```python
from build123d import *

# Parameters (mm, degrees)
SKETCH1_W           = 60
SKETCH1_H           = 100
BOSS_EXTRUDE1_DEPTH = 30
SKETCH2_W           = 60
SKETCH2_H           = 100
BOSS_EXTRUDE2_DEPTH = 30
SKETCH3_W           = 20
SKETCH3_H           = 30
BOSS_EXTRUDE3_DEPTH = 30
SKETCH4_W           = 1.6
SKETCH4_H           = 3
BOSS_EXTRUDE4_DEPTH = 28.4


with BuildPart() as part:
    # Sketch1 → Boss-Extrude1 (new, symmetric)
    with BuildSketch(Plane.XY):
        with Locations((0, -65)):
            Rectangle(SKETCH1_W, SKETCH1_H)
    extrude(amount=BOSS_EXTRUDE1_DEPTH, both=True)



with BuildPart() as body_2:
    # Sketch2 → Boss-Extrude2 (new, symmetric)
    with BuildSketch(Plane.XY):
        with Locations((0, 65)):
            Rectangle(SKETCH2_W, SKETCH2_H)
    extrude(amount=BOSS_EXTRUDE2_DEPTH, both=True)


with BuildPart() as part_1:
    add(part.part)

    add(body_2.part)  # Boss-Extrude3 merges body 2
    # Sketch3 → Boss-Extrude3 (add, symmetric)
    with BuildSketch(Plane.XY):
        Rectangle(SKETCH3_W, SKETCH3_H)
    extrude(amount=BOSS_EXTRUDE3_DEPTH, both=True)

    # Sketch4 → Boss-Extrude4 (add, symmetric)
    with BuildSketch(Plane.XY):
        with Locations((-10.8, -11.9)):
            Rectangle(SKETCH4_W, SKETCH4_H)
    extrude(amount=BOSS_EXTRUDE4_DEPTH, both=True)


solid = part_1.part
```
Read the model definition and answer for the solid it produces. Units are mm, in the model's axes. A direction names the side the tool comes from. Give positions to 0.01 mm unless a question says otherwise; leave off trailing zeros. Order: outer loops, then holes, each group sorted by start corner. A loop starts at its lowest first (then second) coordinate and runs counter-clockwise, first axis right, second up. Notation, with made-up numbers: (-10.5, 20) -> (17.5, 20) arc R9 cw to (17.5, 34) -> close; hole circle Ø11 at (6.5, 50). An arc over 180 degrees is marked (long way). One line per item, written item: value. Start each with the question number.
(1) The part is cut by section B-B (z = 14). Determine the outline of the cut face in (x, y), and give its area (3 significant figures).
(2) The part is cut by section C-C (y = 10). Determine the outline of the cut face in (x, z).
(3) Flat-ended cylindrical pins translate along their axes: P1, Ø3.5, axis at y = -12.5, z = 0, coming from the -X side; P2, Ø0.8, axis at x = -11, y = -11.5, coming from the +Z side; P3, Ø15, axis at y = -2, z = 5.5, coming from the -X side; P4, Ø24, axis at y = 7.5, z = -15, coming from the +X side. Find the tip coordinate at first contact, or state that the pin passes through.
(4) The part is cut by section A-A (x = -19). Determine the outline of the cut face in (y, z).
(5) Straight lines are drawn through the part: L1, parallel to Y at x = -11.5, z = -19.5; L2, parallel to Y at x = 23.5, z = -27.5; L3, parallel to X at y = 10, z = -1. For each, find the intervals that lie inside material, in ascending order.
(6) For a pull along Y with two mould halves and no side action, classify faces 4 (the flat face through (0, 115, 0)), 5 (the flat face through (0, -115, 0)), 6 (the flat face through (30, 64, 0)), 7 (the flat face through (10, 0, 0)) as released by +Y, released by -Y, zero draft, split by the parting line, or undercut.
(7) A tool of negligible diameter and unlimited length cuts with its end or side. For faces 1 (the flat face through (-20, -15, 0)), 2 (the flat face through (20, 15, 0)), 3 (the flat face through (0, 2, -30)), from which of +Z, -Z, +X, -X, +Y, -Y can it reach the whole face along a straight path? Write none if from no direction.
Taken from the geometry:
1. outline: (-30, -115) -> (30, -115) -> (30, -15) -> (10, -15) -> (10, 15) -> (30, 15) -> (30, 115) -> (-30, 115) -> (-30, 15) -> (-10, 15) -> (-10, -10.4) -> (-11.6, -10.4) -> (-11.6, -13.4) -> (-10, -13.4) -> (-10, -15) -> (-30, -15) -> close
1. area: 12,600 mm^2
2. outline: (-10, -30) -> (10, -30) -> (10, 30) -> (-10, 30) -> close
3. P1: x = -11.6
3. P2: z = 28.4
3. P3: x = -10
3. P4: x = 30
4. outline: (-115, -30) -> (-15, -30) -> (-15, 30) -> (-115, 30) -> close; (15, -30) -> (115, -30) -> (115, 30) -> (15, 30) -> close
5. L1: -115 to -15, -13.4 to -10.4, 15 to 115
5. L2: -115 to -15, 15 to 115
5. L3: -10 to 10
6. face 4: released by +Y
6. face 5: released by -Y
6. face 6: zero draft
6. face 7: undercut
7. face 1: +Z, -Z, -X
7. face 2: +Z, -Z, +X
7. face 3: -Z, +X, -X, +Y, -Y
